Source: CAD feature listing. Evaluate the final solid. Frame: model axes, mm. A direction names the side the tool comes from. Give positions to 0.01 mm unless a question says otherwise; leave off trailing zeros. Order: outer loops, then holes, each group sorted by start corner. A loop starts at its lowest first (then second) coordinate and runs counter-clockwise, first axis right, second up.
from build123d import *

# Parameters (mm, degrees)
SKETCH1_W           = 25.4
SKETCH1_H           = 12.7
BOSS_EXTRUDE1_DEPTH = 9.525
SKETCH2_R           = 1.5875
BOSS_EXTRUDE2_DEPTH = 9.525
FILLET1_R           = 4.572


with BuildPart() as part:
    # Sketch1 → Boss-Extrude1 (new body)
    with BuildSketch(Plane(origin=(0, 0, 0), x_dir=(1, 0, 0), z_dir=(0, 1, 0))):
        with Locations((12.7, 6.35)):
            Rectangle(SKETCH1_W, SKETCH1_H)
    extrude(amount=BOSS_EXTRUDE1_DEPTH)

    # Sketch2 → Boss-Extrude2 (add)
    with BuildSketch(Plane.ZY):
        with Locations(Location((-6.35, 4.7625, 0), (0, 0, 180))):
            Circle(SKETCH2_R)
    extrude(amount=BOSS_EXTRUDE2_DEPTH)

    # Fillet1
    fillet1_edges = [part.edges().sort_by_distance(p)[0] for p in [
        (12.7, 9.525, -12.7),
        (12.7, 0, -12.7),
        (12.7, 0, 0),
        (12.7, 9.525, 0),
    ]]
    fillet(fillet1_edges, radius=FILLET1_R)


solid = part.part
1) Reachability of faces 1 (the face through (13, 0, -6)), 2 (the face through (0, 6, -8)) from +Z, -Z, +X, -X, +Y, -Y: full face, straight path, thin tool, end or side. Return the list, or none.
Checks:
face 1: +Z, -Z, +X, -X, -Y
face 2: -X
2) Section query C-C on y = 8.5. Output: boundary loops of the cut face in (x, z), and give its area (3 significant figures).
Checks:
outline: (0, -11.01) - (25.4, -11.01) - (25.4, -1.69) - (0, -1.69) - close
area: 237 mm2
3) Ray query, L1, parallel to X at y = 5.5, z = -9.5; L2, parallel to Y at x = 14, z = -8.25; L3, parallel to Y at x = 13, z = -9.25. Return the intervals inside material, ascending.
Checks:
L1: x = 0 to 25.4
L2: y = 0 to 9.52
L3: y = 0.14 to 9.39
4) First-contact query: pin 1 Ø2 at (x, y) = (7, 3) entering from -Z; pin 2 Ø2 at (y, z) = (4, -2) entering from -X. Flat tips, straight axial feed; report the tip coordinate or a pass-through.
Checks:
pin 1: stops at z = -12.66
pin 2: stops at x = 0
5) Section query A-A on x = 15.5. Output: boundary loops of the cut face in (y, z) (3 decimals).
Checks:
outline: (0, -8.128) arc R4.572 ccw to (4.572, -12.7) - (4.953, -12.7) arc R4.572 ccw to (9.525, -8.128) - (9.525, -4.572) arc R4.572 ccw to (4.953, 0) - (4.572, 0) arc R4.572 ccw to (0, -4.572) - close
6) Section query B-B on z = -6.35. Output: boundary loops of the cut face in (x, y) (3 decimals).
Checks:
outline: (-9.525, 3.175) - (0, 3.175) - (0, 0) - (25.4, 0) - (25.4, 9.525) - (0, 9.525) - (0, 6.35) - (-9.525, 6.35) - close
7) Section query D-D on z = -10.75. Output: boundary loops of the cut face in (x, y), and give its area (3 significant figures).
Checks:
outline: (0, 0.83) - (25.4, 0.83) - (25.4, 8.7) - (0, 8.7) - close
area: 200 mm2
